from build123d import *

# Parameters (mm, degrees)
F0_W     = 577.85
F0_H     = 508
F1_DEPTH = 127
F2_W     = 558.8
F2_H     = 488.95
F3_DEPTH = 120.65
F5_DEPTH = 9.525
F6_R     = 25.4


with BuildPart() as f1:
    # F0 (on Top) → F1 (new body)
    with BuildSketch(Plane.XY):
        with Locations((288.925, -254)):
            Rectangle(F0_W, F0_H)
    extrude(amount=F1_DEPTH)

    # F2 (on face) → F3 (cut)
    with BuildSketch(Plane.XY.offset(127)):
        with Locations((288.925, -254)):
            Rectangle(F2_W, F2_H)
    extrude(amount=-F3_DEPTH, mode=Mode.SUBTRACT)

    # F4 (on face) → F5 (cut, through all)
    with BuildSketch(Plane.XZ.offset(508)):
        Polygon((403.225, 127), (174.625, 127), (206.375, 82.55), (371.475, 82.55), align=None)
    extrude(amount=-F5_DEPTH, mode=Mode.SUBTRACT)

    # F6
    f6_edges = [f1.edges().sort_by_distance(p)[0] for p in [
        (403.225, -503.2375, 127),
        (371.475, -503.2375, 82.55),
        (174.625, -503.2375, 127),
        (206.375, -503.2375, 82.55),
    ]]
    fillet(f6_edges, radius=F6_R)


solid = f1.part
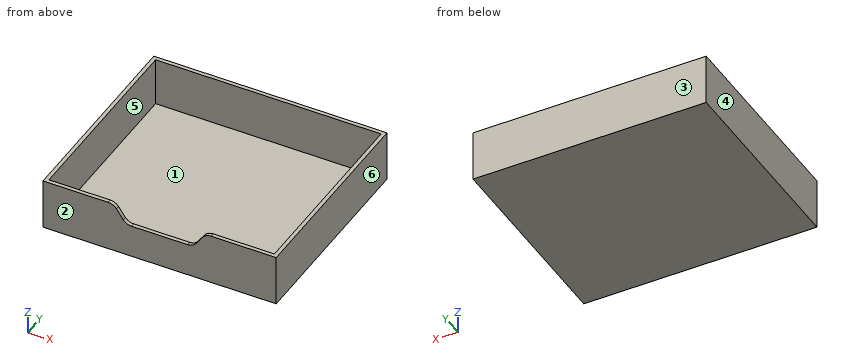
CAD build for the part. Positions are in the model's coordinates, mm. Face numbers are marked on the shaded views. A direction names the side the tool comes from. Give positions to 0.01 mm unless a question says otherwise; leave off trailing zeros. Write each loop counter-clockwise with the first axis right and the second up, starting at its lowest first coordinate (ties: lowest second). Pieces come first, ordered by that corner, then holes. Notation, with made-up numbers: (64, 7) -> (105, 7) arc R17 ccw to (105, 16) -> close; hole circle Ø3 at (63, 41). An arc over 180 degrees is marked (long way). Return JSON: item names as keys, results as strings.
Item 1: Band-saw the part on C-C (y = -175.5). List the corners of the cut face in (x, z) (3 decimals), then the cut area to 3 significant figures.
Answer below:
{"outline": "(0, 0) -> (577.85, 0) -> (577.85, 127) -> (568.325, 127) -> (568.325, 6.35) -> (9.525, 6.35) -> (9.525, 127) -> (0, 127) -> close", "area": "5,970 mm2"}
Item 2: Band-saw the part on A-A (z = 53). List the corners of the cut face in (x, y) (3 decimals).
Answer below:
{"outline": "(0, -508) -> (577.85, -508) -> (577.85, 0) -> (0, 0) -> close; hole (9.525, -498.475) -> (568.325, -498.475) -> (568.325, -9.525) -> (9.525, -9.525) -> close"}
Item 3: Drill centre lines: probe 1 along X at (y, z) = (-171, 96.5) (3 decimals); probe 2 along Y at (x, z) = (474.5, 80) (3 decimals); probe 3 along Z at (x, y) = (543, -320). Where is each one in solid material? Low to high.
Answer below:
{"probe 1": "x = 0 to 9.525, 568.325 to 577.85", "probe 2": "y = -508 to -498.475, -9.525 to 0", "probe 3": "z = 0 to 6.35"}
Item 4: Band-saw the part on B-B (x = 315). List the corners of the cut face in (y, z) (3 decimals), then the cut area to 3 significant figures.
Answer below:
{"outline": "(-508, 0) -> (0, 0) -> (0, 127) -> (-9.525, 127) -> (-9.525, 6.35) -> (-498.475, 6.35) -> (-498.475, 82.55) -> (-508, 82.55) -> close", "area": "5,100 mm2"}
Item 5: Drop a flat-ended pin along its axis: pin 1 (10.5 mm diameter, centred on x = 311.5, y = -501, fed in from +Z). Give the stop position or say it passes through.
Answer below:
{"pin 1": "stops at z = 82.55"}
Item 6: Band-saw the part on D-D (z = 103). List the corners of the cut face in (x, y) (3 decimals).
Answer below:
{"outline": "(0, -508) -> (191.768, -508) -> (191.768, -498.475) -> (9.525, -498.475) -> (9.525, -9.525) -> (568.325, -9.525) -> (568.325, -498.475) -> (386.082, -498.475) -> (386.082, -508) -> (577.85, -508) -> (577.85, 0) -> (0, 0) -> close"}
Item 7: Tool access for the marked faces 5 and 6: list every direction of +Z, -Z, +X, -X, +Y, -Y with a clear straight run to the whole face (end or side of a thin tool).
Answer below:
{"face 5": "+Z", "face 6": "+Z, -Z, +X, +Y, -Y"}
Item 8: Two-plate mould, pull along Y, no slides. Class the marked faces 1, 2, 3 and 4: +Y half, -Y half, draft (parallel to the pull), parting line (faces both ways), or undercut.
Answer below:
{"face 1": "undercut", "face 2": "-Y half", "face 3": "+Y half", "face 4": "draft"}
